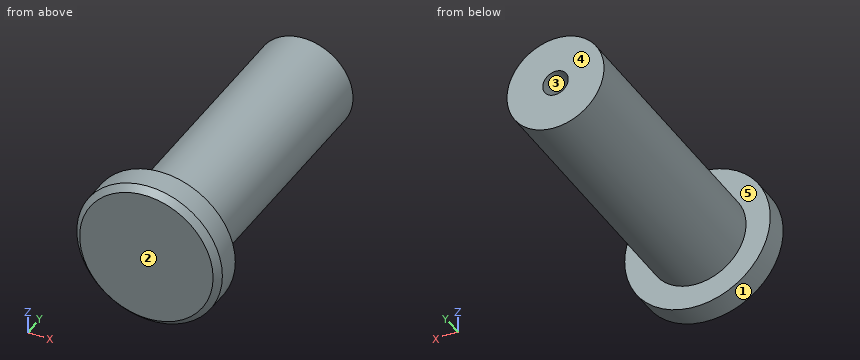
from build123d import *

# Parameters (mm, degrees)
F0_R     = 40
F1_DEPTH = 110
F2_R     = 60
F3_DEPTH = 25
F4_SIZE  = 5
F5_R     = 10.5
F6_DEPTH = 70


with BuildPart() as f1:
    # F0 (on Front) → F1 (new body, symmetric)
    with BuildSketch(Plane.XZ):
        Circle(F0_R)
    extrude(amount=F1_DEPTH, both=True)

    # F2 (on face) → F3 (join)
    with BuildSketch(Plane.XZ.offset(110)):
        Circle(F2_R)
    extrude(amount=F3_DEPTH)

    # F4
    f4_edges = [f1.edges().sort_by_distance(p)[0] for p in [
        (-60, -135, 0),
    ]]
    chamfer(f4_edges, length=F4_SIZE)

    # F5 (on face) → F6 (cut)
    with BuildSketch(Plane(origin=(0, 110, 0), x_dir=(-1, 0, 0), z_dir=(0, 1, 0))):
        Circle(F5_R)
    extrude(amount=-F6_DEPTH, mode=Mode.SUBTRACT)


solid = f1.part
Part model, mm, in its own coordinate system. Face numbers are marked on the shaded views. A direction names the side the tool comes from. Coordinates: 2 decimals unless noted, no trailing zeros. Loops run counter-clockwise (first coordinate to the right, second up) from the corner with the lowest first, then second, coordinate; pieces in that order, holes last. Notation, with made-up numbers: (-34.5, 27) -> (7.5, 27) arc R10 ccw to (7.5, 31) -> close; hole circle Ø10 at (45.5, -38.75). An arc over 180 degrees is marked (long way). Use a Markdown table: item, result. Add a question column.
Item 1: Pull direction Z, two halves, no side cores. Call the marked faces 1, 2 and 3: +Z half, -Z half, draft (parallel to the pull), parting line (faces both ways), or undercut.
Item 2: Band-saw the part on A-A on z = 0. Write the cut outline in (x, y).
Item 3: Flat gauge pins, fed straight in: P1, Ø4, axis at y = -21.5, z = -30.5, coming from the +X side; P2, Ø2, axis at y = -90.5, z = 28, coming from the -X side; P3, Ø5, axis at y = -109.5, z = -26.5, coming from the -X side. Where does each tip first touch, or does it go through?
Item 4: Band-saw the part on B-B on x = 0. Write the cut outline in (y, z).
Item 5: Band-saw the part on C-C on y = 67.5. Write the cut outline in (x, z), plus the area to 3 significant figures.
Item 6: Probe probe 1 along Z at (x, y) = (0, 81); probe 2 along Y at (x, z) = (53, 7); probe 3 along Y at (x, z) = (-43, -39). List the from-to ranges inside material, lowest first.
Item 7: Which spindle directions (+Z, -Z, +X, -X, +Y, -Y) get a long thin tool onto all of the face, cutting with end or side? Do the marked faces 4 and 5. Say none if no direction does.
Item 8: Band-saw the part on D-D on y = -2. Write the cut outline in (x, z).
Geometry says:
| question | item | result |
|---|---|---|
| 1 | face 1 | parting line |
| 1 | face 2 | draft |
| 1 | face 3 | undercut |
| 2 | outline | (-60, -130) -> (-55, -135) -> (55, -135) -> (60, -130) -> (60, -110) -> (40, -110) -> (40, 110) -> (10.5, 110) -> (10.5, 40) -> (-10.5, 40) -> (-10.5, 110) -> (-40, 110) -> (-40, -110) -> (-60, -110) -> close |
| 3 | P1 | x = 28.07 |
| 3 | P2 | x = -29.51 |
| 3 | P3 | x = -54.97 |
| 4 | outline | (-135, -55) -> (-130, -60) -> (-110, -60) -> (-110, -40) -> (110, -40) -> (110, -10.5) -> (40, -10.5) -> (40, 10.5) -> (110, 10.5) -> (110, 40) -> (-110, 40) -> (-110, 60) -> (-130, 60) -> (-135, 55) -> close |
| 5 | outline | circle Ø80 at (0, 0); hole circle Ø21 at (0, 0) |
| 5 | area | 4,680 mm² |
| 6 | probe 1 | -40 to -10.5, 10.5 to 40 |
| 6 | probe 2 | -135 to -110 |
| 6 | probe 3 | -131.95 to -110 |
| 7 | face 4 | +Z, -Z, +X, -X, +Y |
| 7 | face 5 | +Y |
| 8 | outline | circle Ø80 at (0, 0) |
